For this review, take the finished solid that the model builds, in its own axes (mm). A direction names the side the tool comes from. Give positions to 0.01 mm unless a question says otherwise; leave off trailing zeros. Loops run counter-clockwise (first coordinate to the right, second up) from the corner with the lowest first, then second, coordinate; pieces in that order, holes last. Notation, with made-up numbers: (85, -19) -> (142, -19) arc R25 ccw to (142, 4) -> close; hole circle Ø3 at (9, 8.25). An arc over 180 degrees is marked (long way). One line per question, with ' | ' between items. Start each with the question number.
(1) Consider section A-A (z = 0). Write out the cut boundary in (x, y), and give its area (3 significant figures).
(2) Draft analysis for pull direction X (two halves, no side actions). For faces 6 (the flat face through (43, 0, 0)), 7 (the flat face through (53, 12, 16)), 8 (the flat face through (54.129, 5.916, -26.046)), state which applies: +X half, -X half, draft (parallel to the pull), parting line (faces both ways), or undercut.
(3) Wall thickness on probe 1 along X at (y, z) = (17.5, 0); probe 2 along X at (y, z) = (18.5, 16.5); probe 3 along Z at (x, y) = (42, 14.5): over which ranges is each line inside the solid? List them lowest first.
(4) Consider section B-B (x = 0). Write out the cut boundary in (y, z).
(5) Consider section D-D (y = 34.5). Write out the cut boundary in (x, z).
(6) Insertion check: P1, Ø1.5, axis at x = 51, z = 20, coming from the +Y side; P2, Ø20, axis at x = 76.5, z = -18.5, coming from the +Y side; P3, Ø7, axis at x = 55.5, y = 23, coming from the -Z side; P4, Ø3, axis at x = 56, z = -20.5, coming from the -Y side. Each pin has a flat end and moves straight along its axis. Give the tip position at first contact, or say it passes through.
(7) Consider section C-C (y = 5.5). Write out the cut boundary in (x, z).
(8) Tool access review of faces 1 (the flat face through (55, 21, 6)), 2 (the flat face through (56, 21, -6)), 3 (the cylindrical face through (-31.973, 21.748, -1.323)), 4 (the cylindrical face through (5.407, 17.748, 17.169)), 5 (the flat face through (-14, 36, 14)): name each direction out of +Z, -Z, +X, -X, +Y, -Y from which nothing blocks a thin tool from reaching the whole face with its end or side.
from build123d import *

# Parameters (mm, degrees)
SKETCH1_R           = 32
SKETCH1_R_2         = 18
BOSS_EXTRUDE1_DEPTH = 36
SKETCH1_6_R         = 21
SKETCH1_6_R_2       = 12
BOSS_EXTRUDE2_DEPTH = 24
BOSS_EXTRUDE3_DEPTH = 12
BOSS_EXTRUDE4_DEPTH = 36
CUT_EXTRUDE2_DEPTH  = 32


with BuildPart() as part:
    # Sketch1 → Boss-Extrude1 (new body)
    with BuildSketch(Plane(origin=(0, 0, 0), x_dir=(1, 0, 0), z_dir=(0, 1, 0))):
        with Locations(Location((0, 0, 0), (0, 0, 270))):  # turned: the seam where the file's is
            Circle(SKETCH1_R)
        with Locations(Location((0, 0, 0), (0, 0, 270))):  # turned: the seam where the file's is
            Circle(SKETCH1_R_2, mode=Mode.SUBTRACT)
    extrude(amount=BOSS_EXTRUDE1_DEPTH)



with BuildPart() as body_2:
    # Sketch1_6 → Boss-Extrude2 (new body)
    with BuildSketch(Plane(origin=(0, 0, 0), x_dir=(1, 0, 0), z_dir=(0, 1, 0))):
        with Locations(Location((100, 0, 0), (0, 0, 270))):  # turned: the seam where the file's is
            Circle(SKETCH1_6_R)
        with Locations(Location((100, 0, 0), (0, 0, 270))):  # turned: the seam where the file's is
            Circle(SKETCH1_6_R_2, mode=Mode.SUBTRACT)
    extrude(amount=BOSS_EXTRUDE2_DEPTH)


with BuildPart() as part_1:
    add(part.part)

    add(body_2.part)  # Boss-Extrude3 merges body 2
    # Sketch2 → Boss-Extrude3 (add)
    with BuildSketch(Plane(origin=(0, 0, 0), x_dir=(1, 0, 0), z_dir=(0, 1, 0))):
        with BuildLine():
            Line((100, 21), (6.955834404, 31.234858216))
            ThreePointArc((6.955834404, 31.234858216), (32, 0), (6.955834404, -31.234858216))
            Line((6.955834404, -31.234858216), (100, -21))
            ThreePointArc((100, -21), (79, 0), (100, 21))
        make_face()
    extrude(amount=BOSS_EXTRUDE3_DEPTH)

    # Sketch3 → Boss-Extrude4 (add)
    with BuildSketch(Plane(origin=(0, 0, 0), x_dir=(1, 0, 0), z_dir=(0, 1, 0))):
        with BuildLine():
            Line((31.432467291, -6), (79.875388203, -6))
            ThreePointArc((79.875388203, -6), (79, 0), (79.875388203, 6))
            Line((79.875388203, 6), (31.432467291, 6))
            ThreePointArc((31.432467291, 6), (32, 0), (31.432467291, -6))
        make_face()
    extrude(amount=BOSS_EXTRUDE4_DEPTH)

    # Sketch5 → Cut-Extrude2 (cut)
    with BuildSketch(Plane.XY.offset(6)):
        Polygon((79.875388203, 24), (31.432467291, 36), (79.875388203, 36), align=None)
    extrude(amount=-CUT_EXTRUDE2_DEPTH, mode=Mode.SUBTRACT)


solid = part_1.part
A:
1) outline: (-32, 0) -> (-18, 0) -> (-18, 36) -> (-32, 36) -> close; (18, 0) -> (88, 0) -> (88, 24) -> (79, 24) -> (79, 24.22) -> (31.43, 36) -> (18, 36) -> close; (112, 0) -> (121, 0) -> (121, 24) -> (112, 24) -> close | area: 2,850 mm^2
2) face 6: draft | face 7: undercut | face 8: +X half
3) probe 1: x = -32 to -18, 18 to 88, 112 to 121 | probe 2: x = -27.42 to -7.19, 7.19 to 27.42, 87.01 to 112.99 | probe 3: z = -6 to 6
4) outline: (0, -32) -> (36, -32) -> (36, -18) -> (0, -18) -> close; (0, 18) -> (36, 18) -> (36, 32) -> (0, 32) -> close
5) outline: (31.43, -6) -> (37.49, -6) -> (37.49, 6) -> (31.43, 6) arc R32 ccw (long way) to start; hole circle Ø36 at (0, 0)
6) P1: stops at y = 12 | P2: stops at y = 24 | P3: stops at z = -6 | P4: stops at y = 0
7) outline: (6.96, -31.23) -> (100, -21) arc R21 ccw to (100, 21) -> (6.96, 31.23) arc R32 ccw (long way) to start; hole circle Ø36 at (0, 0); hole circle Ø24 at (100, 0)
8) face 1: +Z, +Y | face 2: -Z, +Y | face 3: +Y | face 4: +Y, -Y | face 5: +Z, -Z, +X, -X, +Y
